Autodesk Inventor part; units mm, degrees
ref_plane "YZ Plane" through (0, 0, 0) normal (1, 0, 0) x (0, 1, 0)
ref_plane "XZ Plane" through (0, 0, 0) normal (0, 1, 0) x (-1, 0, 0)
ref_plane "XY Plane" through (0, 0, 0) normal (0, 0, 1) x (1, 0, 0)
sketch "Sketch1" plane through (0, 0, 0) normal (0, 0, 1) x (1, 0, 0)
  line L0 (-13.9366, 26.5) -> (29.645, 26.5)
  line L1 (29.645, 26.5) -> (29.645, -26.5)
  line L2 (29.645, -26.5) -> (-13.9366, -26.5)
  line L3 (-29.645, -12.4581) -> (-29.645, 12.4581)
  line L4 (-29.645, 26.5) -> (29.645, -26.5) construction
  line L5 (29.645, 26.5) -> (-29.645, -26.5) construction
  circle A0 centre (-11.1685, 19.25) radius 7.25 construction
  circle A1 centre (-18.965, 7.68) radius 10.68 construction
  line L6 (-29.645, 7.68) -> (29.645, 7.68) construction
  line L7 (29.645, 0) -> (-29.645, 0) construction
  line L8 (29.645, 26.5) -> (-12.105, 26.5) construction
  line L9 (-16.0003, 24.6552) -> (-26.0827, 15.6424) construction
  line L10 (-13.9366, 26.5) -> (-29.645, 12.4581)
  line L11 (-29.645, -12.4581) -> (-13.9366, -26.5)
  line L12 (-13.9366, 26.5) -> (-13.9366, -26.5) construction
  point P0 (0, 0)
  dimension "d3" = 14.5
  dimension "d4" = 21.36
  dimension "d0" = 59.29
  dimension "d2" = 53
  dimension "d6" = 7.68
  dimension "d7" = 41.75
  dimension "d8" = 12.4581
  dimension "d9" = 12.4581
  dimension "d10" = 43.5816
  dimension "d11" = 59.29
extrude "Extrusion1" add sketch "Sketch1" along normal mid plane 3.17
sketch "Sketch2" plane through (0, 0, 1.585) normal (0, 0, 1) x (1, 0, 0)
  line L0 (-29.645, 12.4581) -> (-29.645, -12.4581)
  line L1 (-13.9366, -26.5) -> (29.645, -26.5)
  line L2 (21.025, -17.51) -> (14.215, -17.51)
  line L3 (14.215, -17.51) -> (14.215, -22.51)
  line L4 (14.215, -22.51) -> (21.025, -22.51)
  line L5 (21.025, -22.51) -> (21.025, -17.51)
  line L6 (21.025, -17.51) -> (14.215, -22.51) construction
  line L7 (14.215, -17.51) -> (21.025, -22.51) construction
  arc A0 (14.215, -17.51) -> (14.215, -22.51) centre (14.215, -20.01) ccw
  arc A1 (21.025, -22.51) -> (21.025, -17.51) centre (21.025, -20.01) ccw
  point P0 (0, 0)
  point P1 (17.62, -20.01)
  dimension "d14" = 6.49
  dimension "d15" = 6.81
  dimension "d16" = 5
  dimension "d17" = 11.81
  dimension "d18" = 43.86
extrude "Extrusion2" cut sketch "Sketch2" against normal through all
pattern_linear "Rectangular Pattern1" count 5 spacing 10 along (0, 1, 0) of "Extrusion2"
sketch "Sketch3" plane through (0, 0, 1.585) normal (0, 0, 1) x (1, 0, 0)
  line L0 (-29.645, 12.4581) -> (-29.645, -12.4581)
  point P0 (0, 0)
  point P1 (-2.785, 0)
  dimension "d24" = 26.86
hole "Hole1" at (-2.785, 0, 1.585) direction (0, 0, -1) diameter 11 end through all counterbore diameter 16.05 counterbore depth 2
sketch "Sketch4" plane through (0, 0, 1.585) normal (0, 0, 1) x (1, 0, 0)
  circle A0 centre (-2.785, 0) radius 8.025
  line L0 (-29.645, 12.4581) -> (-29.645, -12.4581)
  point P0 (0, 0)
  point P1 (-2.785, 21.91)
  point P2 (-2.785, -21.91)
  point P3 (-24.685, 0)
  dimension "d34" = 26.86
  dimension "d35" = 43.82
  dimension "d36" = 21.91
  dimension "d37" = 4.96
  dimension "d38" = 21.9
hole "Hole2" at (-2.785, 21.91, 1.585) at (-2.785, -21.91, 1.585) at (-24.685, 0, 1.585) direction (0, 0, -1) diameter 3 end through all
fillet "Fillet1" radius 7.25 1 edges at (-13.9366, -26.5, 0)
fillet "Fillet2" radius 7.25 1 edges at (-13.9366, 26.5, 0)
fillet "Fillet3" radius 10.68 2 edges at (-29.645, 12.4581, 0) (-29.645, -12.4581, 0)
fillet "Fillet4" radius 4 2 edges at (29.645, -26.5, 0) (29.645, 26.5, 0)
equation "\"d9\" = d8"
properties part number "Threaded Rod Plate" material "Aluminum 6061"
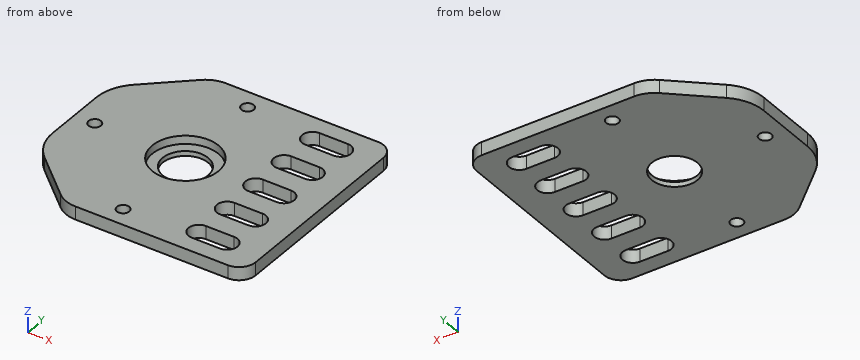
Design review of the part built by this model. Coordinates are the model's own, in mm. Coordinates: 2 decimals unless noted, no trailing zeros. Order: outer loops, then holes, each group sorted by start corner. A loop starts at its lowest first (then second) coordinate and runs counter-clockwise, first axis right, second up. Notation, with made-up numbers: (-0.75, 21) - (53.25, 21) arc R15 cw to (53.25, 40) - close; hole circle Ø8 at (71.5, 15.25). An arc over 180 degrees is marked (long way). Answer in a Markdown table with one row per item.
(1) Consider section A-A on y = 4.5. State the section outline as (x, z) points (3 decimals).
Checked values:
| item | result |
|---|---|
| outline | (-29.645, -1.585) - (-5.947, -1.585) - (-5.947, -0.415) - (-9.43, -0.415) - (-9.43, 1.585) - (-29.645, 1.585) - close; (0.377, -1.585) - (29.645, -1.585) - (29.645, 1.585) - (3.86, 1.585) - (3.86, -0.415) - (0.377, -0.415) - close |
(2) Consider section D-D on z = -1.1. Give the number of separate pieces and of enclosed holes in the cut face, plus the area to 3 significant figures.
Checked values:
| item | result |
|---|---|
| separate pieces | 1 |
| enclosed holes | 9 |
| area | 2,520 mm^2 |
(3) Clearance check with flat-ended pins moving along their axes: pin 1 (9.5 mm diameter, centred on x = -2.785, y = 0, fed in from +Z); pin 2 (5 mm diameter, centred on x = -5.5, y = -3.5, fed in from +Z) (3 decimals). State where each tip first meets the part, or that it passes through.
Checked values:
| item | result |
|---|---|
| pin 1 | through |
| pin 2 | z = -0.415 |
(4) Wall thickness on line 1 along X through (y, z) = (0, 0.3) (3 decimals); line 2 along Y through (x, z) = (14.5, -0.9); line 3 along X through (y, z) = (0, -0.95) (3 decimals): over which ranges is each line inside the solid? List them lowest first. Write a range as from..to.
Checked values:
| item | result |
|---|---|
| line 1 | -29.645..-26.185, -23.185..-10.81, 5.24..11.715, 23.525..29.645 |
| line 2 | -26.5..-22.51, -17.51..-12.51, -7.51..-2.51, 2.49..7.49, 12.49..17.49, 22.49..26.5 |
| line 3 | -29.645..-26.185, -23.185..-8.285, 2.715..11.715, 23.525..29.645 |
(5) Consider section C-C on y = -19. State the section outline as (x, z) points (3 decimals).
Checked values:
| item | result |
|---|---|
| outline | (-22.327, -1.585) - (11.928, -1.585) - (11.928, 1.585) - (-22.327, 1.585) - close; (23.312, -1.585) - (29.645, -1.585) - (29.645, 1.585) - (23.312, 1.585) - close |
(6) Consider section B-B on x = -6. State the section outline as (y, z) points (3 decimals).
Checked values:
| item | result |
|---|---|
| outline | (-26.5, -1.585) - (-4.462, -1.585) - (-4.462, -0.415) - (-7.353, -0.415) - (-7.353, 1.585) - (-26.5, 1.585) - close; (4.462, -1.585) - (26.5, -1.585) - (26.5, 1.585) - (7.353, 1.585) - (7.353, -0.415) - (4.462, -0.415) - close |
